Verification items for the finished model (mm, model axes). A direction names the side the tool comes from. Give positions to 0.01 mm unless a question says otherwise; leave off trailing zeros. Order: outer loops, then holes, each group sorted by start corner. A loop starts at its lowest first (then second) coordinate and runs counter-clockwise, first axis right, second up. Notation, with made-up numbers: (-23, 65) -> (22, 65) arc R12 cw to (22, 88) -> close; hole circle Ø3 at (46.5, 47.5). An arc over 180 degrees is marked (long way). Return JSON: item names as keys, results as strings. Group by question number.
(1) Tool access check on faces 1 (the face through (14, 3.175, 2)), 2 (the face through (-17.46, 4.66, 1.57)), 3 (the face through (12.73, 34.48, 1.57)), 4 (the face through (31, 34.747, 2)), 5 (the face through (0, 2, 2)). Record the directions out of +Z, -Z, +X, -X, +Y, -Y that give a thin tool (end or side, any length) a straight path to the whole face; none if there is none.
(2) Cross-section at C-C on y = 32.5. Enter the section's corners in (x, z) (3 decimals), then the cut area to 3 significant figures.
(3) Cross-section at D-D on y = 19.5. Enter the section's corners in (x, z) (3 decimals), then the cut area to 3 significant figures.
(4) Cross-section at A-A on x = 39. Enter the section's corners in (y, z) (3 decimals), then the cut area to 3 significant figures.
(5) Thickness scan on line 1 along X through (y, z) = (17, 2.7); line 2 along X through (y, z) = (34.5, 2); line 3 along X through (y, z) = (29.5, 2.4). Record the ranges inside material, lowest first.
(6) Depth check by flat-ended pin: pin 1 Ø1.6 at (y, z) = (32, 2) entering from -X; pin 2 Ø1.6 at (x, z) = (13, 1.5) entering from -Y (3 decimals); pin 3 Ø1 at (x, z) = (33, 1.5) entering from -Y. Enter the tip coordinate at first touch or a pass-through.
(7) Release check for a two-part mould opening along X. For faces 6 (the face through (21.612, 32, 2)), 7 (the face through (33, 25.4, 2)), 8 (the face through (-12.7, 2, 2)), 9 (the face through (42.932, 26.355, 1.61)) record: pulls with the +X half, pulls with the -X half, needs draft (parallel to the pull), parting line crosses it, or undercut.
from build123d import *

# Parameters (mm, degrees)
SKETCH1_W           = 19.05
SKETCH1_H           = 5.9944
BOSS_EXTRUDE1_DEPTH = 3.175
FILLET1_R           = 3.175
FILLET2_R           = 3.175


with BuildPart() as part:
    # Sketch1 → Boss-Extrude1 (new body)
    with BuildSketch(Plane.XY):
        with BuildLine():
            Line((0, 3.175), (6.35, 3.175))
            Line((6.35, 3.175), (6.35, 0))
            Line((6.35, 0), (12.087173363, 0))
            Line((12.087173363, 0), (12.087173363, 3.175))
            Line((12.087173363, 3.175), (15.262173363, 3.175))
            ThreePointArc((15.262173363, 3.175), (19.752301423, 5.034871939), (21.612173363, 9.525))
            Line((21.612173363, 9.525), (21.612173363, 25.4))
            Line((21.612173363, 25.4), (43.837173363, 25.4))
            Line((43.837173363, 25.4), (43.837173363, 38.1))
            Line((43.837173363, 38.1), (21.612173363, 38.1))
            ThreePointArc((21.612173363, 38.1), (12.631917242, 34.380256121), (8.912173363, 25.4))
            Line((8.912173363, 25.4), (8.912173363, 10.772098947))
            Line((8.912173363, 10.772098947), (-16.152297099, 6.325593909))
            ThreePointArc((-16.152297099, 6.325593909), (-17.456386706, 4.623315466), (-15.875, 3.175))
            Line((-15.875, 3.175), (-12.7, 3.175))
            Line((-12.7, 3.175), (-12.7, 0))
            Line((-12.7, 0), (0, 0))
            Line((0, 0), (0, 3.175))
        make_face()
        with Locations((31.137173363, 31.75)):
            Rectangle(SKETCH1_W, SKETCH1_H, mode=Mode.SUBTRACT)
    extrude(amount=BOSS_EXTRUDE1_DEPTH)

    # Fillet1
    fillet1_edges = [part.edges().sort_by_distance(p)[0] for p in [
        (8.912173363, 10.772098947, 1.5875),
        (21.612173363, 25.4, 1.5875),
    ]]
    fillet(fillet1_edges, radius=FILLET1_R)

    # Fillet2
    fillet2_edges = [part.edges().sort_by_distance(p)[0] for p in [
        (43.837173363, 38.1, 1.5875),
        (43.837173363, 25.4, 1.5875),
    ]]
    fillet(fillet2_edges, radius=FILLET2_R)


solid = part.part
Verdict:
{
 "1": {"face 1": "+Z, -Z, +X, -Y", "face 2": "+Z, -Z, -X", "face 3": "+Z, -Z, -X, +Y", "face 4": "+Z, -Z", "face 5": "+Z, -Z, -Y"},
 "2": {"outline": "(11.082, 0) -> (21.612, 0) -> (21.612, 3.175) -> (11.082, 3.175) -> close; (40.662, 0) -> (43.837, 0) -> (43.837, 3.175) -> (40.662, 3.175) -> close", "area": "43.5 mm²"},
 "3": {"outline": "(8.912, 0) -> (21.612, 0) -> (21.612, 3.175) -> (8.912, 3.175) -> close", "area": "40.3 mm²"},
 "4": {"outline": "(25.4, 0) -> (28.753, 0) -> (28.753, 3.175) -> (25.4, 3.175) -> close; (34.747, 0) -> (38.1, 0) -> (38.1, 3.175) -> (34.747, 3.175) -> close", "area": "21.3 mm²"},
 "5": {"line 1": "8.91 to 21.61", "line 2": "12.75 to 21.61, 40.66 to 43.84", "line 3": "9.59 to 21.61, 40.66 to 43.84"},
 "6": {"pin 1": "x = 10.31", "pin 2": "y = 3.175", "pin 3": "y = 25.4"},
 "7": {"face 6": "undercut", "face 7": "needs draft", "face 8": "pulls with the -X half", "face 9": "pulls with the +X half"}
}
